from build123d import *

# Parameters (mm, degrees)
F0_W          = 38
F0_H          = 6
F1_DEPTH      = 57.5
F1_DEPTH_BACK = 57.5
F2_R          = 4
F3_DEPTH      = 6
F4_R          = 8
F5_DEPTH      = 39


with BuildPart() as f1:
    # F0 (on Front) → F1 (new body, two sides)
    with BuildSketch(Plane.XZ) as f1_sk:
        Rectangle(F0_W, F0_H)
    extrude(amount=F1_DEPTH)
    extrude(f1_sk.sketch, amount=-F1_DEPTH_BACK)

    # F2 (on face) → F3 (cut)
    with BuildSketch(Plane.XY.offset(3)):
        with Locations((0, 39.5)):
            Circle(F2_R)
        with Locations((0, -39.5)):
            Circle(F2_R)
    extrude(amount=-F3_DEPTH, mode=Mode.SUBTRACT)

    # F4 (on face) → F5 (join)
    with BuildSketch(Plane.XY.offset(3)):
        with Locations((0, 19.5)):
            Circle(F4_R)
    extrude(amount=F5_DEPTH)


solid = f1.part
The model under review builds one solid part; all positions refer to its coordinate system, in mm. Round coordinates to 2 decimals unless told otherwise and drop trailing zeros. Loops run counter-clockwise (first coordinate to the right, second up) from the corner with the lowest first, then second, coordinate; pieces in that order, holes last. Notation, with made-up numbers: M 81,50.5 L 91,50.5 A29 cw 91,87.5 Z; hole C 34,-21.75 d8. An arc over 180 degrees is marked long. Answer as a JSON object with one key per item and string values.
Item 1: For line 1 along Y through (x, z) = (0, 1); line 2 along Y through (x, z) = (1, 0.5); line 3 along Z through (x, y) = (-5, -29), list the stretches that pass through material, from the lowest coordinate up.
Check sheet entries:
{"line 1": "-57.5 to -43.5, -35.5 to 35.5, 43.5 to 57.5", "line 2": "-57.5 to -43.37, -35.63 to 35.63, 43.37 to 57.5", "line 3": "-3 to 3"}
Item 2: The part is to be moulded in two halves that separate along Y. For faces 1 (the face through (7.63, 21.9, 22.23)), 2 (the face through (-0.521, 43.466, 0.042)), 3 (the face through (0, 20, 42)), 4 (the face through (-0.521, -35.534, 0.042)), say which applies: +Y half, -Y half, draft (parallel to the pull), parting line (faces both ways), or undercut.
Check sheet entries:
{"face 1": "parting line", "face 2": "undercut", "face 3": "draft", "face 4": "undercut"}
Item 3: Clearance check with flat-ended pins moving along their axes: P1, Ø8, axis at y = 9.5, z = 5, coming from the +X side; P2, Ø10, axis at x = 11.5, z = 12.5, coming from the -Y side; P3, Ø4, axis at y = 9, z = 9, coming from the +X side; P4, Ø10, axis at x = 6.5, z = 11.5, coming from the +Y side. State where each tip first meets the part, or that it passes through.
Check sheet entries:
{"P1": "x = 19", "P2": "y = 14.84", "P3": "through", "P4": "y = 27.36"}
Item 4: We need section D-D, the plane z = 14.5. State the section outline as (x, y) points.
Check sheet entries:
{"outline": "C 0,19.5 d16"}
Item 5: We need section C-C, the plane y = 19.5. State the section outline as (x, z) points.
Check sheet entries:
{"outline": "M -19,-3 L 19,-3 L 19,3 L 8,3 L 8,42 L -8,42 L -8,3 L -19,3 Z"}
Item 6: We need section B-B, the plane x = 2. State the section outline as (y, z) points.
Check sheet entries:
{"outline": "M -57.5,-3 L -42.96,-3 L -42.96,3 L -57.5,3 Z; M -36.04,-3 L 36.04,-3 L 36.04,3 L 27.25,3 L 27.25,42 L 11.75,42 L 11.75,3 L -36.04,3 Z; M 42.96,-3 L 57.5,-3 L 57.5,3 L 42.96,3 Z"}
Item 7: We need section A-A, the plane y = -39.5. State the section outline as (x, z) points, and give its area (3 significant figures).
Check sheet entries:
{"outline": "M -19,-3 L -4,-3 L -4,3 L -19,3 Z; M 4,-3 L 19,-3 L 19,3 L 4,3 Z", "area": "180 mm2"}
